Verification items for the finished model (mm, model axes). Face numbers are marked on the shaded views. A direction names the side the tool comes from. Round coordinates to 2 decimals unless told otherwise and drop trailing zeros. Loops run counter-clockwise (first coordinate to the right, second up) from the corner with the lowest first, then second, coordinate; pieces in that order, holes last. Notation, with made-up numbers: (50.5, 29.5) - (82.5, 29.5) arc R24 ccw to (82.5, 58.5) - close; hole circle Ø6 at (34, 67). An arc over 180 degrees is marked (long way). Use CSV: the item, a comma, the result in double quotes.
```python
from build123d import *

# Parameters (mm, degrees)
F0_W      = 40
F0_H      = 20
F1_DEPTH  = 5
F2_W      = 40
F2_H      = 6
F3_DEPTH  = 5
F4_R      = 2.75
F5_DEPTH  = 25
F6_W      = 11.2
F6_H      = 6
F7_DEPTH  = 5
F8_R      = 2.6
F9_DEPTH  = 5
F10_R     = 2.6
F11_DEPTH = 4
F12_R     = 1


# Not quite as in the source:
# - a fillet or chamfer that OpenCascade refuses, or shapes differently, is made with other operations: its cross-section is extruded or revolved along the edge and cut away or added
# - a feature names something its author has since deleted; it is built from what else it names


with BuildPart() as f1:
    # F0 (on Top) → F1 (new body)
    with BuildSketch(Plane.XY):
        with Locations((20, 0)):
            Rectangle(F0_W, F0_H)
    extrude(amount=F1_DEPTH)

    # F2 (on face) → F3 (join)
    with BuildSketch(Plane.XY.offset(5)):
        with Locations((20, 0)):
            Rectangle(F2_W, F2_H)
    extrude(amount=F3_DEPTH)

    # F4 (on face) → F5 (cut)
    with BuildSketch(Plane.XY.offset(10)):
        with Locations((10, 0)):
            Circle(F4_R)
    extrude(amount=-F5_DEPTH, mode=Mode.SUBTRACT)

    # F6 (on face) → F7 (cut, through all)
    with BuildSketch(Plane.XY.offset(10)):
        with Locations((28.35, 0)):
            Rectangle(F6_W, F6_H)
    extrude(amount=-F7_DEPTH, mode=Mode.SUBTRACT)

    # F8 (on face) → F9 (cut, through all)
    with BuildSketch(Plane.XY.offset(5)):
        with Locations((28.35, 0)):
            Circle(F8_R)
    extrude(amount=-F9_DEPTH, mode=Mode.SUBTRACT)

    # F10 (on face) → F11 (join)
    with BuildSketch(Plane(origin=(0, 0, 0), x_dir=(0, -1, 0), z_dir=(-1, 0, 0))):
        Polygon((-10, 25), (-10, 5), (-3, 5), (-3, 10), (3, 10), (3, 5), (10, 5), (10, 25), align=None)
        with Locations((0, 15)):
            Circle(F10_R, mode=Mode.SUBTRACT)
        Polygon((-10, 5), (-10, 0), (10, 0), (10, 5), (3, 5), (3, 10), (-3, 10), (-3, 5), align=None)
    extrude(amount=F11_DEPTH)

    # F12
    f12_edges = [f1.edges().sort_by_distance(p)[0] for p in [
        (-2, -10, 25),
        (-2, 10, 25),
        (18, -10, 0),
        (18, 10, 0),
    ]]
    fillet(f12_edges, radius=F12_R)

    # F13: chamfer of 0.5 x 0.2886751346 on 1 edges, made by hand

    # F13_s1 → F13_t2 (revolve, cut)
    with BuildSketch(Plane.XZ):
        Polygon((13.0386751346, 0), (12.75, 0.5), (12.75, 0), align=None)
    revolve(axis=Axis((10, 0, 0), (0, 0, 1)), mode=Mode.SUBTRACT)


solid = f1.part
```
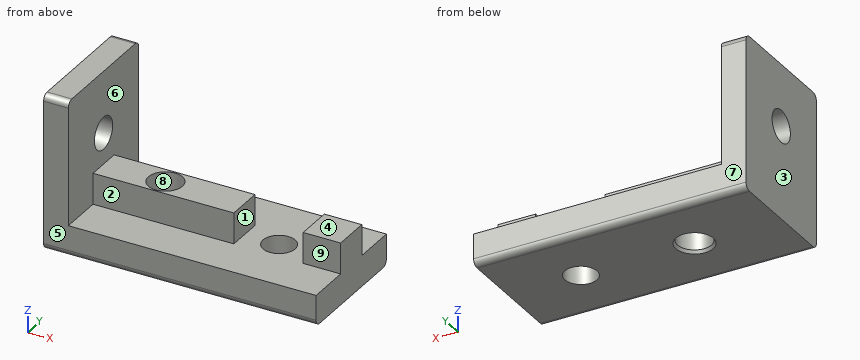
1) Thickness scan on probe 1 along Z at (x, y) = (-1.65, 0); probe 2 along Y at (x, z) = (10, 8); probe 3 along X at (y, z) = (0.5, 9). Record the ranges inside material, lowest first. Write a range as [from, to].
Returned:
probe 1,"z = [0, 12.4], [17.6, 25]"
probe 2,"y = [-3, -2.75], [2.75, 3]"
probe 3,"x = [-4, 7.3], [12.7, 22.75], [33.95, 40]"
2) Cross-section at A-A, the plane x = 28.35. Record the cut outline in (y, z).
Returned:
outline,"(-10, 1) arc R1 ccw to (-9, 0) - (-2.6, 0) - (-2.6, 5) - (-10, 5) - close; (2.6, 0) - (9, 0) arc R1 ccw to (10, 1) - (10, 5) - (2.6, 5) - close"
3) Cross-section at B-B, the plane z = 15. Record the cut outline in (x, y).
Returned:
outline,"(-4, -10) - (0, -10) - (0, -2.6) - (-4, -2.6) - close; (-4, 2.6) - (0, 2.6) - (0, 10) - (-4, 10) - close"
4) Mould release check, pull along Y, two halves, no side actions. Record for the marked faces 6, 7, 8 and 9: +Y half, -Y half, draft (parallel to the pull), parting line (faces both ways), or undercut.
Returned:
face 6,"draft"
face 7,"+Y half"
face 8,"undercut"
face 9,"-Y half"
5) Cross-section at D-D, the plane y = 0. Record the cut outline in (x, z).
Returned:
outline,"(-4, 0) - (6.96, 0) - (7.25, 0.5) - (7.25, 10) - (0, 10) - (0, 12.4) - (-4, 12.4) - close; (-4, 17.6) - (0, 17.6) - (0, 25) - (-4, 25) - close; (12.75, 0.5) - (13.04, 0) - (25.75, 0) - (25.75, 5) - (22.75, 5) - (22.75, 10) - (12.75, 10) - close; (30.95, 0) - (40, 0) - (40, 10) - (33.95, 10) - (33.95, 5) - (30.95, 5) - close"
6) Gauge pin test, flat ends, axial feed: pin 1 Ø1.5 at (x, z) = (37.5, 8.5) entering from +Y; pin 2 Ø1.5 at (x, z) = (11.5, 8) entering from -Y; pin 3 Ø5 at (x, y) = (29.5, -3) entering from +Z; pin 4 Ø1.5 at (x, y) = (29, 0) entering from +Z. Record the tip position at first contact, or that the pin passes through.
Returned:
pin 1,"stops at y = 3"
pin 2,"stops at y = -3"
pin 3,"stops at z = 5"
pin 4,"passes through"
7) Access from +Z, -Z, +X, -X, +Y, -Y to the whole of each face (thin tool, end or side, straight path). Record for the marked faces 1, 2, 3, 4 and 5.
Returned:
face 1,"+Z, +Y, -Y"
face 2,"+Z, +X, -Y"
face 3,"+Z, -Z, -X, +Y, -Y"
face 4,"+Z, +X, +Y, -Y"
face 5,"+Z, -Z, +X, -X, -Y"
8) Cross-section at C-C, the plane z = 5.5. Record the cut outline in (x, y).
Returned:
outline,"(-4, -10) - (0, -10) - (0, -3) - (22.75, -3) - (22.75, 3) - (0, 3) - (0, 10) - (-4, 10) - close; (33.95, -3) - (40, -3) - (40, 3) - (33.95, 3) - close; hole circle Ø5.5 at (10, 0)"
